Study the drawing (mm; zero at the part's minimum x, y, z) and answer. Round coordinates to 2 decimals unless told otherwise and drop trailing zeros. Write each loop counter-clockwise with the first axis right and the second up, starting at its lowest first coordinate (ties: lowest second). Pieces come first, ordered by that corner, then holes.
(1) This flat-tipped pin is pushed along its axis until it touches: pin 1 Ø0.9 at (x, y) = (3.5, 2) entering from +Z. Where does it stop, or does it pass through?
(2) A cutting plane is placed at A-A, the plane z = 3.75. Give the vertices of the cut face in (x, y).
(3) Find the intervals of material crossed by probe 1 along X at (y, z) = (1.4, 2.25); probe 2 along X at (y, z) = (1.9, 1.4); probe 3 along X at (y, z) = (0.6, 1), in increasing order.
(4) A cutting plane is placed at B-B, the plane y = 1.7. Give the vertices of the cut face in (x, z), and give its area (3 significant figures).
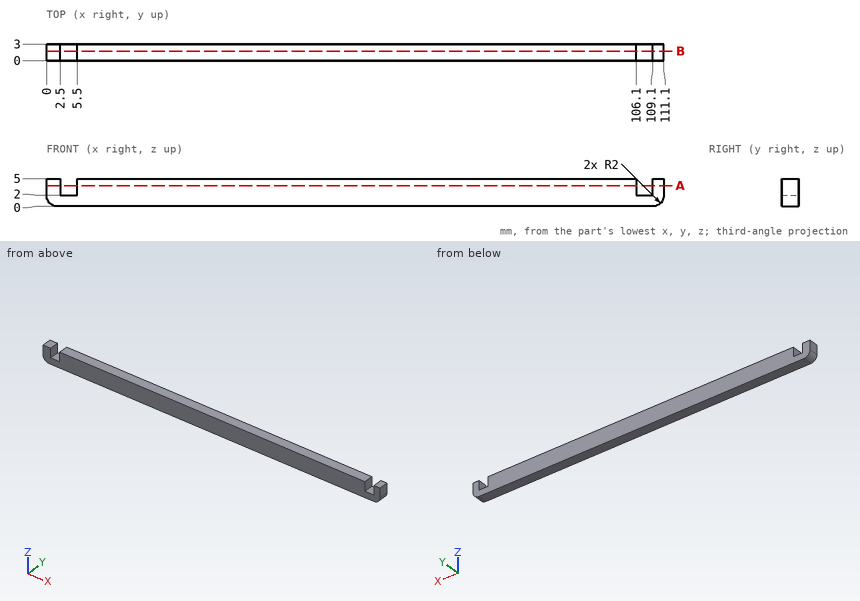
Solutions:
1. pin 1: stops at z = 2
2. outline: (0, 0) - (2.5, 0) - (2.5, 3) - (0, 3) - close; (5.5, 0) - (106.1, 0) - (106.1, 3) - (5.5, 3) - close; (109.1, 0) - (111.1, 0) - (111.1, 3) - (109.1, 3) - close
3. probe 1: x = 0 to 2.5, 5.5 to 106.1, 109.1 to 111.1
3. probe 2: x = 0.09 to 111.01
3. probe 3: x = 0.27 to 110.83
4. outline: (0, 2) arc R2 ccw to (2, 0) - (109.1, 0) arc R2 ccw to (111.1, 2) - (111.1, 5) - (109.1, 5) - (109.1, 2) - (106.1, 2) - (106.1, 5) - (5.5, 5) - (5.5, 2) - (2.5, 2) - (2.5, 5) - (0, 5) - close
4. area: 536 mm2
